Geometry: final body of the model. Coordinates: model frame, mm. A direction names the side the tool comes from. Give positions to 0.01 mm unless a question says otherwise; leave off trailing zeros. Loops run counter-clockwise (first coordinate to the right, second up) from the corner with the lowest first, then second, coordinate; pieces in that order, holes last. Notation, with made-up numbers: (8, 30) -> (49, 30) arc R14 ccw to (49, 37) -> close; hole circle Ø6 at (27.25, 21.5). An arc over 180 degrees is marked (long way). One line per question, with ' | ' between items. Start each with the question number.
Item 1: Section D-D on z = 1.25. Return loops of the section in (x, y) (1 decimal).
Item 2: Section A-A on y = 0. Return loops of the section in (x, z).
Item 3: Material intervals for line 1 along Z through (x, y) = (4.5, 0); line 2 along Z through (x, y) = (-1.25, 0); line 3 along Z through (x, y) = (-3, 2.5), sorted ascending. Write a range as [from, to].
Item 4: Section C-C on x = -1.5. Return loops of the section in (y, z) (3 decimals).
Item 5: Pin query (flat end, axial travel): P1, Ø1.7, axis at y = 0, z = 3.81, coming from the -X side; P2, Ø1.7, axis at y = 1, z = -2.5, coming from the -X side. Return the tip coordinate at first contact, or that it passes through.
Item 6: Set-up query: faces 1 (the flat face through (1, 0, 7.62)), 2 (the flat face through (-2, 0, 0)). Return all of +Z, -Z, +X, -X, +Y, -Y with unobstructed straight access to the full face (end or side cutting, diameter ignored); none if empty.
Item 7: Mould query, pull axis Z, two halves, no side actions, for faces 3 (the cylindrical face through (1.602, -0.187, 5.233)), 4 (the flat face through (0.737, 0, -2)), 5 (the flat face through (4, 0, -3.302)). Classes: released by +Z, released by -Z, zero draft, split by the parting line, or undercut.
from build123d import *

# Parameters (mm, degrees)
F0_W     = 6.35
F0_H     = 6.35
F1_DEPTH = 3.302
F2_W     = 11.1252
F2_H     = 7.62
F3_DEPTH = 3.175
F4_R     = 1.4351
F5_DEPTH = 11.1262
F6_SIZE  = 1.5875


with BuildPart() as f1:
    # F0 (on Top) → F1 (new body)
    with BuildSketch(Plane.XY):
        with Locations((3.9116, 0)):
            Rectangle(F0_W, F0_H)
    extrude(amount=-F1_DEPTH)

    # F2 (on Front) → F3 (join, symmetric)
    with BuildSketch(Plane.XZ):
        with Locations((1.524, 3.81)):
            Rectangle(F2_W, F2_H)
    extrude(amount=F3_DEPTH, both=True)

    # F4 (on face) → F5 (cut, through all)
    with BuildSketch(Plane.YZ.offset(7.0866)):
        with Locations((0, 3.81)):
            Circle(F4_R)
    extrude(amount=-F5_DEPTH, mode=Mode.SUBTRACT)

    # F6
    f6_edges = [f1.edges().sort_by_distance(p)[0] for p in [
        (-4.0386, -3.175, 3.81),
        (-4.0386, 3.175, 3.81),
    ]]
    chamfer(f6_edges, length=F6_SIZE)


solid = f1.part
Result sheet:
1) outline: (-4, -1.6) -> (-2.5, -3.2) -> (7.1, -3.2) -> (7.1, 3.2) -> (-2.5, 3.2) -> (-4, 1.6) -> close
2) outline: (-4.04, 0) -> (0.74, 0) -> (0.74, -3.3) -> (7.09, -3.3) -> (7.09, 2.37) -> (-4.04, 2.37) -> close; (-4.04, 5.25) -> (7.09, 5.25) -> (7.09, 7.62) -> (-4.04, 7.62) -> close
3) line 1: z = [-3.3, 2.37], [5.25, 7.62] | line 2: z = [0, 2.37], [5.25, 7.62] | line 3: z = [0, 7.62]
4) outline: (-3.175, 0) -> (3.175, 0) -> (3.175, 7.62) -> (-3.175, 7.62) -> close; hole circle Ø2.87 at (0, 3.81)
5) P1: passes through | P2: stops at x = 0.74
6) face 1: +Z, +X, -X, +Y, -Y | face 2: -Z, -X, +Y, -Y
7) face 3: undercut | face 4: zero draft | face 5: released by -Z
